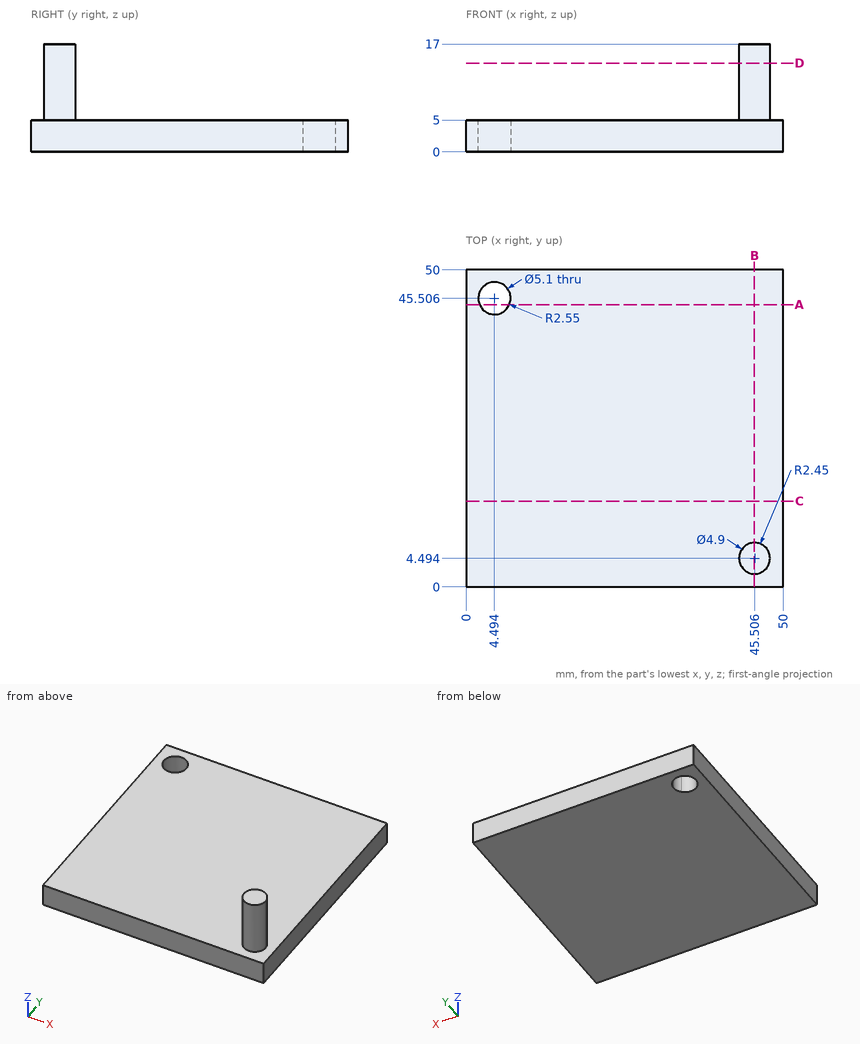
Geometry check sheet. Reference: drawing and pictorial views, mm from the part's lowest x, y, z. Coordinates: 2 decimals unless noted, no trailing zeros. Order: outer loops, then holes, each group sorted by start corner. A loop starts at its lowest first (then second) coordinate and runs counter-clockwise, first axis right, second up. Notation, with made-up numbers: (85, 40) -> (126, 40) arc R13 cw to (126, 46) -> close; hole circle Ø7 at (20, 40.5). An arc over 180 degrees is marked (long way). Write item = value, one per line. Start each with the question number.
1) Cross-section at B-B (x = 45.5). Enter the section's corners in (y, z).
2) Material ranges on L1, parallel to Z at x = 47, y = 7; L2, parallel to X at y = 46, z = 4.75; L3, parallel to X at y = 44, z = 1.75, recorded low to high.
3) Cross-section at C-C (y = 13.5). Enter the section's corners in (x, z), then the cut area to 3 significant figures.
4) Cross-section at D-D (z = 14). Enter the section's corners in (x, y).
5) Cross-section at A-A (y = 44.5). Enter the section's corners in (x, z).
6) Go/stop test with flat-tipped pins: P1, Ø8, axis at x = 42, z = 10.5, coming from the +Y side; P2, Ø1, axis at x = 44, z = 8.5, coming from the -Y side; P3, Ø15, axis at x = 25, y = 19.5, coming from the +Z side. Record where each tip stops, or that it passes through.
Ans:
q1.outline = (0, 0) -> (50, 0) -> (50, 5) -> (6.94, 5) -> (6.94, 17) -> (2.04, 17) -> (2.04, 5) -> (0, 5) -> close
q2.L1 = 0 to 5
q2.L2 = 0 to 1.99, 7 to 50
q2.L3 = 0 to 2.44, 6.55 to 50
q3.outline = (0, 0) -> (50, 0) -> (50, 5) -> (0, 5) -> close
q3.area = 250 mm²
q4.outline = circle Ø4.9 at (45.51, 4.49)
q5.outline = (0, 0) -> (2.15, 0) -> (2.15, 5) -> (0, 5) -> close; (6.84, 0) -> (50, 0) -> (50, 5) -> (6.84, 5) -> close
q6.P1 = 6.94
q6.P2 = 2.26
q6.P3 = 5
